Geometry: final body of the model. Coordinates: model frame, mm. A direction names the side the tool comes from. Coordinates: 2 decimals unless noted, no trailing zeros. Order: outer loops, then holes, each group sorted by start corner. A loop starts at its lowest first (then second) coordinate and runs counter-clockwise, first axis right, second up. Notation, with made-up numbers: M 9,62 L 38,62 A27 ccw 38,100 Z; hole C 21,-36.5 d7. An arc over 180 degrees is marked long. Write item = value, one per line.
from build123d import *

# Parameters (mm, degrees)
SKETCH1_W           = 660.4
SKETCH1_H           = 25.4
BOSS_EXTRUDE1_DEPTH = 25.4
SHELL1_T            = -3.175


with BuildPart() as part:
    # Sketch1 → Boss-Extrude1 (new body, symmetric)
    with BuildSketch(Plane(origin=(0, 0, 0), x_dir=(1, 0, 0), z_dir=(0, 1, 0))):
        Rectangle(SKETCH1_W, SKETCH1_H)
    extrude(amount=BOSS_EXTRUDE1_DEPTH, both=True)

    # Shell1
    shell1_openings = [part.faces().sort_by_distance(p)[0] for p in [
        (-330.2, 0, 0),
        (330.2, 0, 0),
    ]]
    offset(amount=SHELL1_T, openings=shell1_openings, kind=Kind.INTERSECTION)


solid = part.part
1) Set-up query: faces 1 (the face through (-5, 0, 9.525)), 2 (the face through (-5, 25.4, 0)). Return all of +Z, -Z, +X, -X, +Y, -Y with unobstructed straight access to the full face (end or side cutting, diameter ignored); none if empty.
Numbers:
face_1 = +X, -X
face_2 = +Z, -Z, +X, -X, +Y
2) Pin query (flat end, axial travel): pin 1 (8 mm diameter, centred on y = -14, z = -8, fed in from -X). Return the tip coordinate at first contact, or that it passes through.
Numbers:
pin_1 = -330.2
3) Mould query, pull axis Y, two halves, no side actions, for faces 3 (the face through (-5, -22.225, 0)), 4 (the face through (-5, 0, -12.7)), 5 (the face through (-5, -25.4, 0)). Classes: pulls with the +Y half, pulls with the -Y half, needs draft (parallel to the pull), parting line crosses it, or undercut.
Numbers:
face_3 = undercut
face_4 = needs draft
face_5 = pulls with the -Y half
4) Section C-C, the plane x = 160. Return loops of the section in (y, z) (3 decimals), and give its area (3 significant figures).
Numbers:
outline = M -25.4,-12.7 L 25.4,-12.7 L 25.4,12.7 L -25.4,12.7 Z; hole M -22.225,-9.525 L 22.225,-9.525 L 22.225,9.525 L -22.225,9.525 Z
area = 444 mm²
5) Line query: L1, parallel to Y at x = -237, z = -2.25 (3 decimals); L2, parallel to Z at x = -74, y = -15 (3 decimals). Output: solid intervals per line, ascending.
Numbers:
L1 = -25.4 to -22.225, 22.225 to 25.4
L2 = -12.7 to -9.525, 9.525 to 12.7
6) Section A-A, the plane z = 2. Return loops of the section in (x, y) (3 decimals).
Numbers:
outline = M -330.2,-25.4 L 330.2,-25.4 L 330.2,-22.225 L -330.2,-22.225 Z; M -330.2,22.225 L 330.2,22.225 L 330.2,25.4 L -330.2,25.4 Z
7) Section B-B, the plane y = -14.5. Return loops of the section in (x, z) (3 decimals).
Numbers:
outline = M -330.2,-12.7 L 330.2,-12.7 L 330.2,-9.525 L -330.2,-9.525 Z; M -330.2,9.525 L 330.2,9.525 L 330.2,12.7 L -330.2,12.7 Z
